Could you check a few things on this model? Use its own coordinates, in mm. Face numbers are marked on the shaded views. Round coordinates to 2 decimals unless told otherwise and drop trailing zeros. Order: outer loops, then holes, each group sorted by start corner. A loop starts at its lowest first (then second) coordinate and runs counter-clockwise, first axis right, second up.
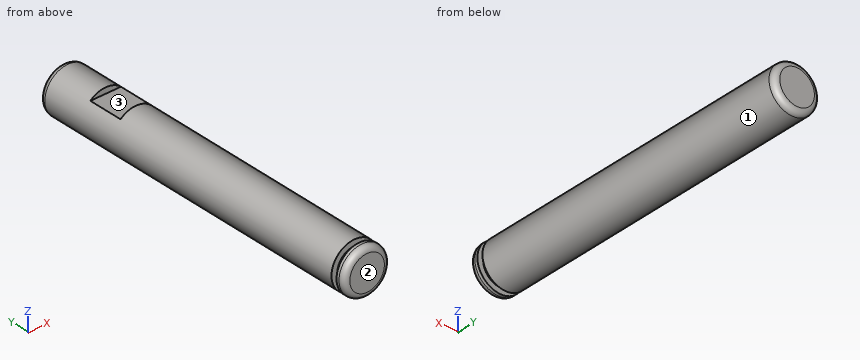
```python
from build123d import *

# Parameters (mm, degrees)
FILLET1_R          = 0.5
CUT_EXTRUDE1_START = 1.5
SKETCH2_W          = 4
SKETCH2_H          = 3
CUT_EXTRUDE1_DEPTH = 29.881943651


with BuildPart() as part:
    # Sketch1 → Revolve1 (revolve)
    with BuildSketch(Plane.XY, mode=Mode.PRIVATE) as revolve1_sk:
        Polygon((-2, 0), (0, 0), (0, 30.25), (-2, 30.25), (-2, 1.25), (-1.5, 1.25), (-1.5, 0.75), (-2, 0.75), align=None)
    revolve(revolve1_sk.sketch.rotate(Axis((0, 0, 0), (0, 1, 0)), 270), axis=Axis((0, 0, 0), (0, 1, 0)))

    # Fillet1
    fillet1_edges = [part.edges().sort_by_distance(p)[0] for p in [
        (0, 30.25, 2),
        (0, 0, 2),
    ]]
    fillet(fillet1_edges, radius=FILLET1_R)

    # Sketch2 → Cut-Extrude1 (cut, through all)
    with BuildSketch(Plane.XY.offset(CUT_EXTRUDE1_START)):
        with Locations((0, 24.5)):
            Rectangle(SKETCH2_W, SKETCH2_H)
    extrude(amount=CUT_EXTRUDE1_DEPTH, mode=Mode.SUBTRACT)


solid = part.part
```
Q1. Imagine slicing it at A-A, the plane x = 0. Please give me the cut outline in (y, z), then the cut area to 3 significant figures.
Q2. Imagine slicing it at B-B, the plane y = 16. Please give me the cut outline in (x, z), then the cut area to 3 significant figures.
Q3. For P1, Ø1.5, axis at x = 1, y = 26, coming from the -Z side; P2, Ø1.3, axis at x = -0.5, y = 25, coming from the +Z side, each with a flat end and sliding along its axis, tell me the tip position at first contact or that it passes through.
Q4. I need wall thicknesses on L1, parallel to Y at x = -1.55, z = 0.25; L2, parallel to X at y = 5.5, z = -1.5; L3, parallel to Y at x = 1.25, z = 1.2. Which ranges of each line are inside material? Lowest first, please.
Q5. We'd pull the mould along Y, two halves only. Please class the marked faces 1, 2 and 3: released by +Y, released by -Y, zero draft, split by the parting line, or undercut.
Filled in:
1. outline: (0, -1.5) arc R0.5 ccw to (0.5, -2) - (0.75, -2) - (0.75, -1.5) - (1.25, -1.5) - (1.25, -2) - (29.75, -2) arc R0.5 ccw to (30.25, -1.5) - (30.25, 1.5) arc R0.5 ccw to (29.75, 2) - (26, 2) - (26, 1.5) - (23, 1.5) - (23, 2) - (1.25, 2) - (1.25, 1.5) - (0.75, 1.5) - (0.75, 2) - (0.5, 2) arc R0.5 ccw to (0, 1.5) - close
1. area: 119 mm2
2. outline: circle Ø4 at (0, 0)
2. area: 12.6 mm2
3. P1: stops at z = -1.98
3. P2: stops at z = 1.5
4. L1: y = 0 to 0.75, 1.25 to 30.25
4. L2: x = -1.32 to 1.32
4. L3: y = 0.06 to 0.75, 1.25 to 30.19
5. face 1: zero draft
5. face 2: released by -Y
5. face 3: undercut
